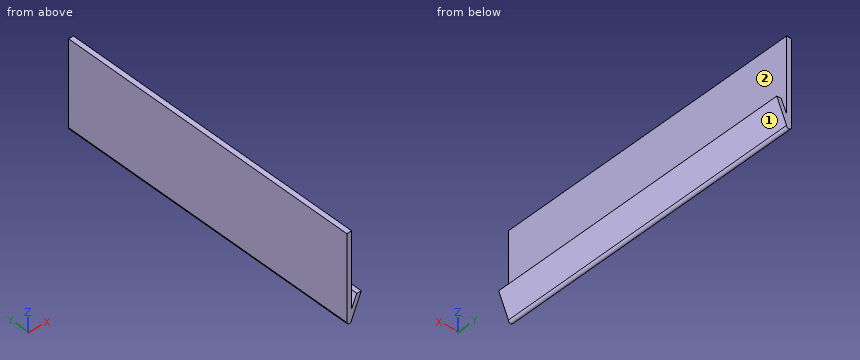
```python
from build123d import *

# Parameters (mm, degrees)
F1_DEPTH = 25.4


with BuildPart() as f1:
    # F0 (on Front) → F1 (new body)
    with BuildSketch(Plane.XZ):
        with BuildLine():
            Line((0, 0), (0, 5.9944))
            Line((0, 5.9944), (-0.390362, 5.977479))
            Line((-0.390362, 5.977479), (-0.390362, -0.856854))
            ThreePointArc((-0.390362, -0.856854), (-0.205291, -1.052327), (0, -0.878212))
            Line((0, -0.878212), (0.784725, 0.96267))
            Line((0.784725, 0.96267), (0.420264, 0.96267))
            Line((0.420264, 0.96267), (0, 0))
        make_face()
    extrude(amount=F1_DEPTH)


solid = f1.part
```
Part model, mm, in its own coordinate system. Face numbers are marked on the shaded views. A direction names the side the tool comes from. Round coordinates to 2 decimals unless told otherwise and drop trailing zeros. Order: outer loops, then holes, each group sorted by start corner. A loop starts at its lowest first (then second) coordinate and runs counter-clockwise, first axis right, second up. Notation, with made-up numbers: M 89.5,16.25 L 147.5,16.25 A16 cw 147.5,20.25 Z; hole C 10,37 d6. An arc over 180 degrees is marked long. Put each result on its own line as item: value. Start each with the question number.
1. Tool access for the marked faces 1 and 2: list every direction of +Z, -Z, +X, -X, +Y, -Y with a clear straight run to the whole face (end or side of a thin tool).
2. Drop a flat-ended pin along its axis: pin 1 (1.5 mm diameter, centred on y = -12, z = 0, fed in from +X). Give the stop position or say it passes through.
3. Slice it at C-C on x = 0.6. List the corners of the cut face in (y, z), then the cut area to 3 significant figures.
4. Slice it at A-A on z = 0.25. List the corners of the cut face in (x, y), then the cut area to 3 significant figures.
5. Slice it at B-B on y = -22. List the corners of the cut face in (x, z).
6. Drill centre lines: probe 1 along X at (y, z) = (-4, 2.5); probe 2 along X at (y, z) = (-9, 0.5); probe 3 along Z at (x, y) = (0.1, -12.5). Where is each one in solid material? Low to high. Write a range as [from, to].
7. Slice it at D-D on z = 5.5. List the corners of the cut face in (x, y).
Findings:
1. face 1: -Z, +X, +Y, -Y
1. face 2: +Z, +Y, -Y
2. pin 1: x = 0.69
3. outline: M -25.4,0.53 L 0,0.53 L 0,0.96 L -25.4,0.96 Z
3. area: 11.0 mm2
4. outline: M -0.39,-25.4 L 0,-25.4 L 0,0 L -0.39,0 Z; M 0.11,-25.4 L 0.48,-25.4 L 0.48,0 L 0.11,0 Z
4. area: 19.4 mm2
5. outline: M -0.39,-0.86 A0.2 ccw 0,-0.88 L 0.78,0.96 L 0.42,0.96 L 0,0 L 0,5.99 L -0.39,5.98 Z
6. probe 1: [-0.39, 0]
6. probe 2: [-0.39, 0], [0.22, 0.59]
6. probe 3: [-0.64, 0.23]
7. outline: M -0.39,-25.4 L 0,-25.4 L 0,0 L -0.39,0 Z
